The model under review builds one solid part; all positions refer to its coordinate system, in mm. Face numbers are marked on the shaded views. A direction names the side the tool comes from. Give positions to 0.01 mm unless a question says otherwise; leave off trailing zeros. Order: outer loops, then holes, each group sorted by start corner. A loop starts at its lowest first (then second) coordinate and runs counter-clockwise, first axis right, second up. Notation, with made-up numbers: (41.5, -1.75) - (92.5, -1.75) arc R22 cw to (92.5, 36.25) - close; hole circle Ø6 at (-6, -26.5). An arc over 180 degrees is marked (long way). Answer as CSV lines item,"result". Start each with the question number.
from build123d import *

# Parameters (mm, degrees)
F1_DEPTH = 2


with BuildPart() as f1:
    # F0 (on Top) → F1 (new body)
    with BuildSketch(Plane.XY):
        Polygon((17.362918, -22.817224), (3.905775, 14.67053), (-16.825457, -1.721608), (0.091206, 0.211725), align=None)
        with BuildLine():
            ThreePointArc((-4.499081, 4.477946), (-4.520667, 4.532407), (-4.541067, 4.587323))
            Line((-4.541067, 4.587323), (-5.173952, 4.919177))
            Line((-5.173952, 4.919177), (-5.217277, 5.745873))
            Line((-5.217277, 5.745873), (-4.622547, 6.142063))
            ThreePointArc((-4.622547, 6.142063), (-4.608, 6.198811), (-4.592224, 6.25523))
            Line((-4.592224, 6.25523), (-4.90918, 6.895706))
            Line((-4.90918, 6.895706), (-4.458311, 7.589984))
            Line((-4.458311, 7.589984), (-3.74429, 7.560935))
            ThreePointArc((-3.74429, 7.560935), (-3.699165, 7.598294), (-3.65324, 7.634665))
            Line((-3.65324, 7.634665), (-3.533201, 8.339123))
            Line((-3.533201, 8.339123), (-2.760354, 8.635791))
            Line((-2.760354, 8.635791), (-2.199773, 8.192599))
            ThreePointArc((-2.199773, 8.192599), (-2.141307, 8.1963), (-2.082775, 8.198731))
            Line((-2.082775, 8.198731), (-1.571591, 8.698092))
            Line((-1.571591, 8.698092), (-0.771967, 8.483833))
            Line((-0.771967, 8.483833), (-0.57895, 7.795782))
            ThreePointArc((-0.57895, 7.795782), (-0.529475, 7.764411), (-0.480692, 7.731973))
            Line((-0.480692, 7.731973), (0.226382, 7.835498))
            Line((0.226382, 7.835498), (0.747352, 7.192153))
            Line((0.747352, 7.192153), (0.499081, 6.522054))
            ThreePointArc((0.499081, 6.522054), (0.520667, 6.467593), (0.541067, 6.412677))
            Line((0.541067, 6.412677), (1.173952, 6.080823))
            Line((1.173952, 6.080823), (1.217277, 5.254127))
            Line((1.217277, 5.254127), (0.622547, 4.857937))
            ThreePointArc((0.622547, 4.857937), (0.608, 4.801189), (0.592224, 4.74477))
            Line((0.592224, 4.74477), (0.90918, 4.104294))
            Line((0.90918, 4.104294), (0.458311, 3.410016))
            Line((0.458311, 3.410016), (-0.25571, 3.439065))
            ThreePointArc((-0.25571, 3.439065), (-0.300835, 3.401706), (-0.34676, 3.365335))
            Line((-0.34676, 3.365335), (-0.466799, 2.660877))
            Line((-0.466799, 2.660877), (-1.239646, 2.364209))
            Line((-1.239646, 2.364209), (-1.800227, 2.807401))
            ThreePointArc((-1.800227, 2.807401), (-1.858693, 2.8037), (-1.917225, 2.801269))
            Line((-1.917225, 2.801269), (-2.428409, 2.301908))
            Line((-2.428409, 2.301908), (-3.228033, 2.516167))
            Line((-3.228033, 2.516167), (-3.42105, 3.204218))
            ThreePointArc((-3.42105, 3.204218), (-3.470525, 3.235589), (-3.519308, 3.268027))
            Line((-3.519308, 3.268027), (-4.226382, 3.164502))
            Line((-4.226382, 3.164502), (-4.747352, 3.807847))
            Line((-4.747352, 3.807847), (-4.499081, 4.477946))
        make_face(mode=Mode.SUBTRACT)
        with BuildLine():
            ThreePointArc((2.880692, 4.731973), (2.929475, 4.764411), (2.97895, 4.795782))
            Line((2.97895, 4.795782), (3.171967, 5.483833))
            Line((3.171967, 5.483833), (3.971591, 5.698092))
            Line((3.971591, 5.698092), (4.482775, 5.198731))
            ThreePointArc((4.482775, 5.198731), (4.541307, 5.1963), (4.599773, 5.192599))
            Line((4.599773, 5.192599), (5.160354, 5.635791))
            Line((5.160354, 5.635791), (5.933201, 5.339123))
            Line((5.933201, 5.339123), (6.05324, 4.634665))
            ThreePointArc((6.05324, 4.634665), (6.099165, 4.598294), (6.14429, 4.560935))
            Line((6.14429, 4.560935), (6.858311, 4.589984))
            Line((6.858311, 4.589984), (7.30918, 3.895706))
            Line((7.30918, 3.895706), (6.992224, 3.25523))
            ThreePointArc((6.992224, 3.25523), (7.008, 3.198811), (7.022547, 3.142063))
            Line((7.022547, 3.142063), (7.617277, 2.745873))
            Line((7.617277, 2.745873), (7.573952, 1.919177))
            Line((7.573952, 1.919177), (6.941067, 1.587323))
            ThreePointArc((6.941067, 1.587323), (6.920667, 1.532407), (6.899081, 1.477946))
            Line((6.899081, 1.477946), (7.147352, 0.807847))
            Line((7.147352, 0.807847), (6.626382, 0.164502))
            Line((6.626382, 0.164502), (5.919308, 0.268027))
            ThreePointArc((5.919308, 0.268027), (5.870525, 0.235589), (5.82105, 0.204218))
            Line((5.82105, 0.204218), (5.628033, -0.483833))
            Line((5.628033, -0.483833), (4.828409, -0.698092))
            Line((4.828409, -0.698092), (4.317225, -0.198731))
            ThreePointArc((4.317225, -0.198731), (4.258693, -0.1963), (4.200227, -0.192599))
            Line((4.200227, -0.192599), (3.639646, -0.635791))
            Line((3.639646, -0.635791), (2.866799, -0.339123))
            Line((2.866799, -0.339123), (2.74676, 0.365335))
            ThreePointArc((2.74676, 0.365335), (2.700835, 0.401706), (2.65571, 0.439065))
            Line((2.65571, 0.439065), (1.941689, 0.410016))
            Line((1.941689, 0.410016), (1.49082, 1.104294))
            Line((1.49082, 1.104294), (1.807776, 1.74477))
            ThreePointArc((1.807776, 1.74477), (1.792, 1.801189), (1.777453, 1.857937))
            Line((1.777453, 1.857937), (1.182723, 2.254127))
            Line((1.182723, 2.254127), (1.226048, 3.080823))
            Line((1.226048, 3.080823), (1.858933, 3.412677))
            ThreePointArc((1.858933, 3.412677), (1.879333, 3.467593), (1.900919, 3.522054))
            Line((1.900919, 3.522054), (1.652648, 4.192153))
            Line((1.652648, 4.192153), (2.173618, 4.835498))
            Line((2.173618, 4.835498), (2.880692, 4.731973))
        make_face(mode=Mode.SUBTRACT)
    extrude(amount=F1_DEPTH)


solid = f1.part
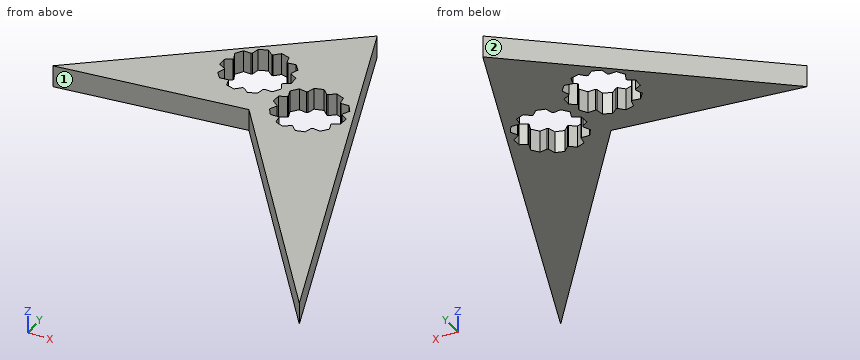
Item 1: Machinability: for the marked faces 1 and 2, which of the approach directions +Z, -Z, +X, -X, +Y, -Y give a long, thin tool a straight path to every point of the face, cutting with its end or side? Answer none if there is none.
Item 2: Take a section at C-C on x = -7. Write out the cut boundary in (y, z), and give its area (3 significant figures).
Item 3: For line 1 along X through (y, z) = (4.5, 1.1); line 2 along X through (y, z) = (7, 0.4); line 3 along Y through (x, z) = (0, 1.9), list the stretches that pass through material, from the lowest coordinate up.
Item 4: Take a section at A-A on z = 1.45. Count the separate pieces of the cut face and the enclosed holes in it, and give its area (3 significant figures).
Item 5: Take a section at B-B on y = -2.5. Write out the cut boundary in (x, z) (3 decimals), and give its area (3 significant figures).
Item 6: Clearance check with a flat-ended pin moving along its axis: pin 1 (1 mm diameter, centred on x = 2, y = 4.5, fed in from +Z). State where the tip first meets the part, or that it passes through.
Data:
1,face 1,"+Z, -Z, -Y"
1,face 2,"+Z, -Z, -X, +Y"
2,outline,"(-0.6, 0) - (6.05, 0) - (6.05, 2) - (-0.6, 2) - close"
2,area,"13.3 mm^2"
3,line 1,"x = -8.96 to -4.51, 0.71 to 1.9, 6.92 to 7.56"
3,line 2,"x = -5.8 to -4.84, 0.68 to 6.66"
3,line 3,"y = 0.2 to 3.43, 7.8 to 11.58"
4,separate pieces,"1"
4,enclosed holes,"2"
4,area,"229 mm^2"
5,outline,"(2.125, 0) - (10.07, 0) - (10.07, 2) - (2.125, 2) - close"
5,area,"15.9 mm^2"
6,pin 1,"stops at z = 2"
